Answer from the drawing. Dimensions are ordinates in mm from the lowest x, y and z of the part. Round coordinates to 2 decimals unless told otherwise and drop trailing zeros. Loops run counter-clockwise (first coordinate to the right, second up) from the corner with the lowest first, then second, coordinate; pieces in that order, holes last. Notation, with made-up numbers: M 0,73.5 L 8,73.5 A25 cw 8,86.5 Z; hole C -18.75,57 d8. An arc over 180 degrees is marked long. Answer as a JSON object with one key per item and string values.
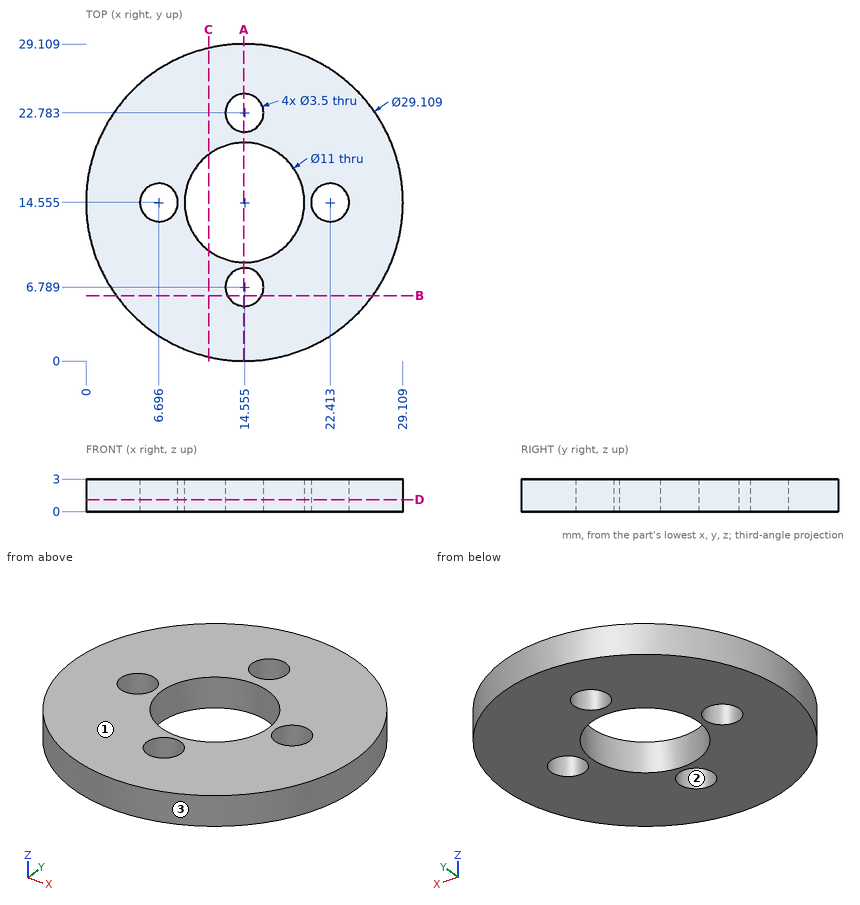
Item 1: Straight lines are drawn through the part: line 1 (X direction, y = 14, z = 1.85) (1 decimal); line 2 (X direction, y = 15.25, z = 1.9); line 3 (X direction, y = 12.5, z = 0.55) (1 decimal). For each, find the intervals that lie inside material, in ascending order.
Values follow:
{"line 1": "0 to 5, 8.4 to 9.1, 20 to 20.8, 24.1 to 29.1", "line 2": "0.02 to 5.09, 8.3 to 9.1, 20.01 to 20.81, 24.02 to 29.09", "line 3": "0.1 to 9.5, 19.7 to 29"}
Item 2: The part is cut by section A-A (x = 14.5). Give the vertices of the cut face in (y, z) (1 decimal).
Values follow:
{"outline": "M 0,0 L 5,0 L 5,3 L 0,3 Z; M 8.5,0 L 9.1,0 L 9.1,3 L 8.5,3 Z; M 20.1,0 L 21,0 L 21,3 L 20.1,3 Z; M 24.5,0 L 29.1,0 L 29.1,3 L 24.5,3 Z"}
Item 3: Determine the mould class of the marked faces 1, 2 and 3 for opening direction Y: released by +Y, released by -Y, zero draft, split by the parting line, or undercut.
Values follow:
{"face 1": "zero draft", "face 2": "undercut", "face 3": "split by the parting line"}
Item 4: The part is cut by section B-B (y = 6). Give the vertices of the cut face in (x, z).
Values follow:
{"outline": "M 2.78,0 L 12.99,0 L 12.99,3 L 2.78,3 Z; M 16.12,0 L 26.33,0 L 26.33,3 L 16.12,3 Z"}
Item 5: The part is cut by section D-D (z = 1.1). Give the number of separate pieces and of enclosed holes in the cut face, then the cut area to 3 significant figures.
Values follow:
{"separate pieces": "1", "enclosed holes": "5", "area": "532 mm^2"}
Item 6: The part is cut by section C-C (x = 11.25). Give the vertices of the cut face in (y, z).
Values follow:
{"outline": "M 0.38,0 L 10.16,0 L 10.16,3 L 0.38,3 Z; M 18.95,0 L 28.73,0 L 28.73,3 L 18.95,3 Z"}
